from build123d import *

# Parameters (mm, degrees)
F0_W     = 16.002
F0_H     = 11.1125
F1_DEPTH = 76.2
F0_R     = 9.017
F2_DEPTH = 10.0076
F3_R     = 9.9695
F4_DEPTH = 25.4


# Not quite as in the source:
# - a feature names something its author has since deleted; it is built from what else it names


with BuildPart() as f1:
    # F0 (on Top) → F1 (new body)
    with BuildSketch(Plane.XY):
        Polygon((-215.5320961376, 0), (-215.5320961376, 38.263771664), (-215.5320961376, 88.9), (-231.5340961376, 88.9), (-231.5340961376, 39.535600692), (-231.5340961376, 0), align=None)
        with Locations((-223.5330961376, -5.55625)):
            Rectangle(F0_W, F0_H)
    extrude(amount=F1_DEPTH)

    # F0 (on Top) → F2 (join)
    with BuildSketch(Plane.XY):
        with BuildLine():
            ThreePointArc((-210.8337106802, 109.7300639993), (-210.8332497742, 109.7925312439), (-210.8330961376, 109.855))
            ThreePointArc((-210.8330961376, 109.855), (-210.8331549592, 109.8936531274), (-210.8333314233, 109.9323058968))
            ThreePointArc((-210.8333314233, 109.9323058968), (-210.8336216962, 109.8311851368), (-210.8337106802, 109.7300639993))
        make_face()
        with BuildLine():
            ThreePointArc((-210.8337106802, 109.7300639993), (-210.8336216962, 109.8311851368), (-210.8333314233, 109.9323058968))
            ThreePointArc((-210.8333314233, 109.9323058968), (-223.438898877, 122.5546506596), (-236.2303167947, 110.12068324))
            ThreePointArc((-236.2303167947, 110.12068324), (-236.2290424274, 109.8342939205), (-236.229382634, 109.5479019679))
            ThreePointArc((-236.229382634, 109.5479019679), (-223.4420019429, 97.1553267031), (-210.8337106802, 109.7300639993))
        make_face()
        with Locations((-223.5330961376, 109.855)):
            Circle(F0_R, mode=Mode.SUBTRACT)
        with BuildLine():
            ThreePointArc((-191.660374853, 69.9817506227), (-205.7887196825, 87.6651452552), (-210.8337106802, 109.7300639993))
            ThreePointArc((-210.8337106802, 109.7300639993), (-223.4420019429, 97.1553267031), (-236.229382634, 109.5479019679))
            ThreePointArc((-236.229382634, 109.5479019679), (-241.3359242696, 87.5526791762), (-255.4702109751, 69.9433483413))
            ThreePointArc((-255.4702109751, 69.9433483413), (-242.6773531137, 70.1074060375), (-236.2330961376, 59.055))
            ThreePointArc((-236.2330961376, 59.055), (-238.6417428115, 51.6133572568), (-244.9540483765, 46.9944370399))
            ThreePointArc((-244.9540483765, 46.9944370399), (-237.2361698926, 45.078438676), (-231.5340961376, 39.535600692))
            Line((-231.5340961376, 39.535600692), (-231.5340961376, 88.9))
            Line((-231.5340961376, 88.9), (-215.5320961376, 88.9))
            Line((-215.5320961376, 88.9), (-215.5320961376, 38.263771664))
            ThreePointArc((-215.5320961376, 38.263771664), (-209.5064918471, 44.6635464864), (-200.94875069, 46.6710551745))
            ThreePointArc((-200.94875069, 46.6710551745), (-209.9310054796, 63.7559929971), (-191.660374853, 69.9817506227))
        make_face()
        with BuildLine():
            ThreePointArc((-236.229382634, 109.5479019679), (-236.2290424274, 109.8342939205), (-236.2303167947, 110.12068324))
            ThreePointArc((-236.2303167947, 110.12068324), (-236.2330792473, 109.8342873368), (-236.229382634, 109.5479019679))
        make_face()
        with BuildLine():
            ThreePointArc((-185.4330961376, 59.055), (-187.0992037982, 65.343339991), (-191.660374853, 69.9817506227))
            ThreePointArc((-191.660374853, 69.9817506227), (-209.9310054796, 63.7559929971), (-200.94875069, 46.6710551745))
            ThreePointArc((-200.94875069, 46.6710551745), (-199.8363704021, 46.5607848043), (-198.7350651606, 46.3692744277))
            ThreePointArc((-198.7350651606, 46.3692744277), (-189.3682517748, 49.8643796022), (-185.4330961376, 59.055))
        make_face()
        with Locations((-198.1330961376, 59.055)):
            Circle(F0_R, mode=Mode.SUBTRACT)
        with BuildLine():
            ThreePointArc((-257.5728060865, 68.3633517337), (-256.5112816453, 69.1397405149), (-255.4702109751, 69.9433483413))
            ThreePointArc((-255.4702109751, 69.9433483413), (-256.5625194428, 69.2079256882), (-257.5728060865, 68.3633517337))
        make_face()
        with BuildLine():
            ThreePointArc((-236.2330961376, 59.055), (-242.6773531137, 70.1074060375), (-255.4702109751, 69.9433483413))
            ThreePointArc((-255.4702109751, 69.9433483413), (-256.5112816453, 69.1397405149), (-257.5728060865, 68.3633517337))
            ThreePointArc((-257.5728060865, 68.3633517337), (-260.7702508926, 54.4537211227), (-249.0179411736, 46.3552834158))
            ThreePointArc((-249.0179411736, 46.3552834158), (-247.0076603385, 46.8126151022), (-244.9540483765, 46.9944370399))
            ThreePointArc((-244.9540483765, 46.9944370399), (-238.6417428115, 51.6133572568), (-236.2330961376, 59.055))
        make_face()
        with Locations((-248.9330961376, 59.055)):
            Circle(F0_R, mode=Mode.SUBTRACT)
        with BuildLine():
            ThreePointArc((-198.7350651606, 46.3692744277), (-199.8363704021, 46.5607848043), (-200.94875069, 46.6710551745))
            ThreePointArc((-200.94875069, 46.6710551745), (-199.8485569009, 46.4713918382), (-198.7350651606, 46.3692744277))
        make_face()
        Polygon((-215.5320961376, 0), (-215.5320961376, 38.263771664), (-215.5320961376, 88.9), (-231.5340961376, 88.9), (-231.5340961376, 39.535600692), (-231.5340961376, 0), align=None)
        with BuildLine():
            ThreePointArc((-249.0179411736, 46.3552834158), (-246.9599430632, 46.5092171649), (-244.9540483765, 46.9944370399))
            ThreePointArc((-244.9540483765, 46.9944370399), (-247.0076603385, 46.8126151022), (-249.0179411736, 46.3552834158))
        make_face()
        with Locations((-223.5330961376, -5.55625)):
            Rectangle(F0_W, F0_H)
    extrude(amount=F2_DEPTH)

    # F3 (on face) → F4 (cut)
    with BuildSketch(Plane(origin=(-231.5340961376, 0, 0), x_dir=(0, -1, 0), z_dir=(-1, 0, 0))):
        with BuildLine():
            ThreePointArc((-26.4295804615, 38.3289644541), (-2.3509786782, 42.6501406146), (11.1125, 22.225))
            Line((11.1125, 22.225), (11.1125, 76.2))
            Line((11.1125, 76.2), (-88.9, 76.2))
            Line((-88.9, 76.2), (-88.9, 10.0076))
            ThreePointArc((-88.9, 10.0076), (-55.490267729, 19.3717854622), (-26.4295804615, 38.3289644541))
        make_face()
        with Locations((-11.1125, 22.225)):
            Circle(F3_R)
        with BuildLine():
            Line((11.1125, 0), (11.1125, 22.225))
            ThreePointArc((11.1125, 22.225), (4.6029482119, 6.5095517881), (-11.1125, 0))
            Line((-11.1125, 0), (0, 0))
            Line((0, 0), (11.1125, 0))
        make_face()
    extrude(amount=-F4_DEPTH, mode=Mode.SUBTRACT)


solid = f1.part
Here's how the part is built. I have some questions about the finished solid (model axes, mm). A direction names the side the tool comes from. Coordinates: 2 decimals unless noted, no trailing zeros. Loops run counter-clockwise (first coordinate to the right, second up) from the corner with the lowest first, then second, coordinate; pieces in that order, holes last. Notation, with made-up numbers: (-28.75, 67) -> (-0.75, 67) arc R37 ccw to (-0.75, 106) -> close; hole circle Ø4 at (22, -26). An arc over 180 degrees is marked (long way). Use one line per item in the form item = value. Start each with the question number.
(1) Will these pins go through, and if not, where does the flat tip stop? pin 1 (6 mm diameter, centred on x = -217.5, y = 9.5, fed in from +Z); pin 2 (1.5 mm diameter, centred on x = -197.5, y = 44, fed in from -Z); pin 3 (2 mm diameter, centred on y = 15.5, z = 6.5, fed in from +X); pin 4 (4 mm diameter, centred on y = 82, z = 5, fed in from +X).
(2) If we section it at B-B (z = 18): Please give me the cut outline in (x, y).
(3) If we section it at C-C (y = 63.5): Please give me the cut outline in (x, z), then the cut area to 3 significant figures.
(4) Please list where these lines run through material, in increasing order: line 1 along X through (y, z) = (46.5, 14.5); line 2 along X through (y, z) = (54.5, 5); line 3 along Z through (x, y) = (-189.5, 65.5).
(5) If we section it at A-A (x = -226): Give the number of separate pieces and of enclosed holes in the cut face, then the cut area to 3 significant figures.
(6) If we section it at D-D (x = -204.5): Please give me the cut outline in (y, z).
(7) On a 3-axis mill with a long thin cutter (end or side, diameter ignored), from which of +Z, -Z, +X, -X, +Y, -Y can I reach the whole of each face in a straight line? I mean faces 4 (the face through (-224, 68, 0)), 5 (the face through (-215.532, 27, 17)), 6 (the face through (-241.198, 87.84, 4.934)), 7 (the face through (-237.33, 45.13, 4.93)), 8 (the face through (-231.534, 28, 22)). Say none if no direction works.
(8) We'd pull the mould along X, two halves only. Please class faces 1 (the face through (-215, 77, 10.008)), 2 (the face through (-205.65, 87.38, 4.93)), 3 (the face through (-209.614, 44.601, 4.934)): pulls with the +X half, pulls with the -X half, needs draft (parallel to the pull), parting line crosses it, or undercut.
Verdict:
q1.pin_1 = 44.45
q1.pin_2 = through
q1.pin_3 = -215.53
q1.pin_4 = -201.22
q2.outline = (-231.53, -10.71) -> (-215.53, -10.71) -> (-215.53, 2.08) -> (-231.53, 2.08) -> close; (-231.53, 20.14) -> (-215.53, 20.14) -> (-215.53, 58.64) -> (-231.53, 58.64) -> close
q3.outline = (-260.83, 0) -> (-256.78, 0) -> (-256.78, 10.01) -> (-260.83, 10.01) -> close; (-241.09, 0) -> (-205.98, 0) -> (-205.98, 10.01) -> (-215.53, 10.01) -> (-215.53, 16.1) -> (-231.53, 16.1) -> (-231.53, 10.01) -> (-241.09, 10.01) -> close; (-190.29, 0) -> (-186.24, 0) -> (-186.24, 10.01) -> (-190.29, 10.01) -> close
q3.area = 530 mm²
q4.line_1 = -231.53 to -215.53
q4.line_2 = -260.79 to -256.72, -241.15 to -205.92, -190.35 to -186.28
q4.line_3 = 0 to 10.01
q5.separate_pieces = 2
q5.enclosed_holes = 1
q5.area = 2,540 mm²
q6.outline = (46.48, 0) -> (52.67, 0) -> (52.67, 10.01) -> (46.48, 10.01) -> close; (65.44, 0) -> (85.17, 0) -> (85.17, 10.01) -> (65.44, 10.01) -> close
q7.face_4 = -Z, +X, -X, +Y, -Y
q7.face_5 = +Z, +X, -Y
q7.face_6 = +Z, -Z, -X, +Y
q7.face_7 = +Z, -Z, -Y
q7.face_8 = +Z, -X, -Y
q8.face_1 = needs draft
q8.face_2 = pulls with the +X half
q8.face_3 = undercut
